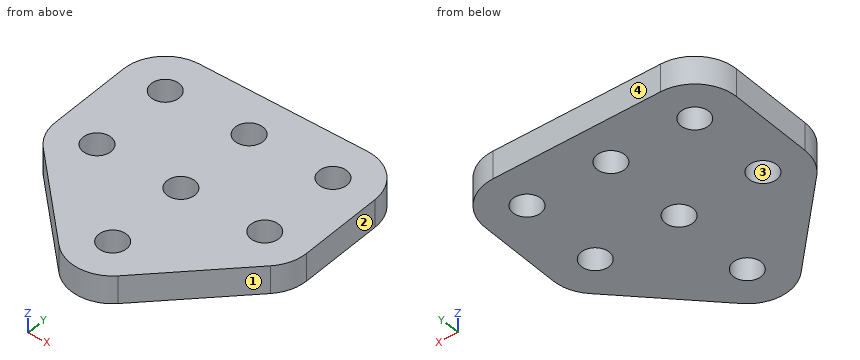
```python
from build123d import *

# Parameters (mm, degrees)
MODEL_R                 = 1.5
SALIENTE_EXTRUIR1_DEPTH = 3


with BuildPart() as part:
    # Model → Saliente-Extruir1 (new body)
    with BuildSketch(Plane.XY):
        with BuildLine():
            Line((174.227054575, 213.178720063), (174.227054575, 204.178720063))
            ThreePointArc((174.227054575, 204.178720063), (174.569596678, 202.456644617), (175.545074059, 200.996739548))
            Line((175.545074059, 200.996739548), (184.545074059, 191.996739548))
            ThreePointArc((184.545074059, 191.996739548), (187.727054575, 190.678720063), (190.90903509, 191.996739548))
            Line((190.90903509, 191.996739548), (199.90903509, 200.996739548))
            ThreePointArc((199.90903509, 200.996739548), (200.884512471, 202.456644617), (201.227054575, 204.178720063))
            Line((201.227054575, 204.178720063), (201.227054575, 213.178720063))
            ThreePointArc((201.227054575, 213.178720063), (199.90903509, 216.360700578), (196.727054575, 217.678720063))
            Line((196.727054575, 217.678720063), (178.727054575, 217.678720063))
            ThreePointArc((178.727054575, 217.678720063), (175.545074059, 216.360700578), (174.227054575, 213.178720063))
        make_face()
        with Locations((187.727054575, 204.178720063)):
            Circle(MODEL_R, mode=Mode.SUBTRACT)
        with Locations((178.727054575, 204.178720063)):
            Circle(MODEL_R, mode=Mode.SUBTRACT)
        with Locations((187.727054575, 213.178720063)):
            Circle(MODEL_R, mode=Mode.SUBTRACT)
        with Locations((178.727054575, 213.178720063)):
            Circle(MODEL_R, mode=Mode.SUBTRACT)
        with Locations((196.727054575, 213.178720063)):
            Circle(MODEL_R, mode=Mode.SUBTRACT)
        with Locations((187.727054575, 195.178720063)):
            Circle(MODEL_R, mode=Mode.SUBTRACT)
        with Locations((196.727054575, 204.178720063)):
            Circle(MODEL_R, mode=Mode.SUBTRACT)
    extrude(amount=SALIENTE_EXTRUIR1_DEPTH)


solid = part.part
```
Geometry check sheet. Reference: the model listing, model coordinates, mm. Face numbers are marked on the shaded views. Give positions to 0.01 mm unless a question says otherwise; leave off trailing zeros. Loops run counter-clockwise (first coordinate to the right, second up) from the corner with the lowest first, then second, coordinate; pieces in that order, holes last. Notation, with made-up numbers: M 88.25,85 L 128.25,85 A22 ccw 128.25,94 Z; hole C -8.5,22 d11. An arc over 180 degrees is marked long. Write item = value, one per line.
(1) Release check for a two-part mould opening along Y. For the marked faces 1, 2, 3 and 4 record: released by +Y, released by -Y, zero draft, split by the parting line, or undercut.
Answer below:
face_1 = released by -Y
face_2 = zero draft
face_3 = undercut
face_4 = released by +Y
(2) Sectioned sample at C-C, the plane x = 182.5. Record the cut outline in (y, z).
Answer below:
outline = M 194.04,0 L 217.68,0 L 217.68,3 L 194.04,3 Z
(3) Gauge pin test, flat end, axial feed: pin 1 Ø6 at (x, y) = (196, 214) entering from +Z. Record the tip position at first contact, or that the pin passes through.
Answer below:
pin_1 = 3
(4) Sectioned sample at B-B, the plane z = 1.4. Record the cut outline in (x, y).
Answer below:
outline = M 174.23,204.18 A4.5 ccw 175.55,201 L 184.55,192 A4.5 ccw 190.91,192 L 199.91,201 A4.5 ccw 201.23,204.18 L 201.23,213.18 A4.5 ccw 196.73,217.68 L 178.73,217.68 A4.5 ccw 174.23,213.18 Z; hole C 178.73,204.18 d3; hole C 178.73,213.18 d3; hole C 187.73,195.18 d3; hole C 187.73,204.18 d3; hole C 187.73,213.18 d3; hole C 196.73,204.18 d3; hole C 196.73,213.18 d3
(5) Sectioned sample at A-A, the plane x = 197.25. Record the cut outline in (y, z), plus the area to 3 significant figures.
Answer below:
outline = M 198.34,0 L 202.77,0 L 202.77,3 L 198.34,3 Z; M 205.58,0 L 211.77,0 L 211.77,3 L 205.58,3 Z; M 214.58,0 L 217.65,0 L 217.65,3 L 214.58,3 Z
area = 41.1 mm2
(6) Sectioned sample at D-D, the plane x = 194.25. Record the cut outline in (y, z).
Answer below:
outline = M 195.34,0 L 217.68,0 L 217.68,3 L 195.34,3 Z
(7) Material ranges on line 1 (Y direction, x = 177.75, z = 2.15); line 2 (Y direction, x = 187.75, z = 1.4); line 3 (X direction, y = 204.5, z = 1), recorded low to high. Write a range as [from, to].
Answer below:
line_1 = [198.79, 203.04], [205.32, 212.04], [214.32, 217.57]
line_2 = [190.68, 193.68], [196.68, 202.68], [205.68, 211.68], [214.68, 217.68]
line_3 = [174.23, 177.26], [180.19, 186.26], [189.19, 195.26], [198.19, 201.23]
